```python
from build123d import *

# Parameters (mm, degrees)
SALIENTE_EXTRUIR1_DEPTH = 2
CROQUIS3_R              = 3.575
CROQUIS3_R_2            = 2.575
SALIENTE_EXTRUIR2_DEPTH = 5


with BuildPart() as part:
    # Croquis1 → Saliente-Extruir1 (new body)
    with BuildSketch(Plane(origin=(0, 0, 0), x_dir=(1, 0, 0), z_dir=(0, 1, 0))):
        with BuildLine():
            Line((-3, 13.162446581), (-4.5, 0))
            Line((-4.5, 0), (-3, -13.162446581))
            ThreePointArc((-3, -13.162446581), (0, -13.5), (3, -13.162446581))
            Line((3, -13.162446581), (4.5, 0))
            Line((4.5, 0), (3, 13.162446581))
            ThreePointArc((3, 13.162446581), (0, 13.5), (-3, 13.162446581))
        make_face()
    extrude(amount=SALIENTE_EXTRUIR1_DEPTH)

    # Croquis3 → Saliente-Extruir2 (add)
    with BuildSketch(Plane(origin=(0, 2, 0), x_dir=(1, 0, 0), z_dir=(0, 1, 0))):
        with Locations(Location((0, 0, 0), (0, 0, 270))):
            Circle(CROQUIS3_R)
        with Locations(Location((0, 0, 0), (0, 0, 270))):
            Circle(CROQUIS3_R_2, mode=Mode.SUBTRACT)
    extrude(amount=SALIENTE_EXTRUIR2_DEPTH)


solid = part.part
```
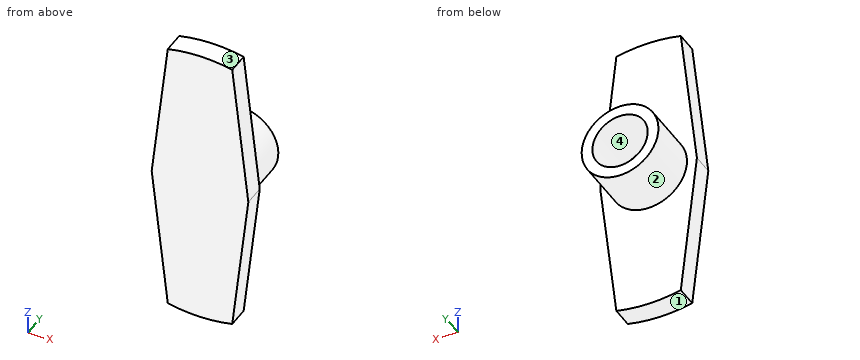
Input: part model. Units: mm. Frame: model coordinates. Face numbers are marked on the shaded views. Give positions to 0.01 mm unless a question says otherwise; leave off trailing zeros. Order: outer loops, then holes, each group sorted by start corner. A loop starts at its lowest first (then second) coordinate and runs counter-clockwise, first axis right, second up. Notation, with made-up numbers: (26, 66) - (38, 66) arc R18 cw to (38, 86) - close; hole circle Ø3 at (19, 59.25). An arc over 180 degrees is marked (long way). Use a Markdown table: item, result.
(1) Section query B-B (y = 3.25). Output: boundary loops of the cut face in (x, z) (3 decimals).
Computed values:
| item | result |
|---|---|
| outline | circle Ø7.15 at (0, 0); hole circle Ø5.15 at (0, 0) |
(2) Line query: line 1 (X direction, y = 4.3, z = 0) (3 decimals); line 2 (Y direction, x = -1.75, z = 12.5); line 3 (Z direction, x = 2, y = 3.5). Output: solid intervals per line, ascending. Write a range as from..to.
Computed values:
| item | result |
|---|---|
| line 1 | x = -3.575..-2.575, 2.575..3.575 |
| line 2 | y = 0..2 |
| line 3 | z = -2.96..-1.62, 1.62..2.96 |
(3) Section query D-D (z = 3). Output: boundary loops of the cut face in (x, y).
Computed values:
| item | result |
|---|---|
| outline | (-4.16, 0) - (4.16, 0) - (4.16, 2) - (1.94, 2) - (1.94, 7) - (-1.94, 7) - (-1.94, 2) - (-4.16, 2) - close |
(4) Draft query along Z for the marked faces 1, 2, 3 and 4. Return one class per face: released by +Z, released by -Z, zero draft, split by the parting line, or undercut.
Computed values:
| item | result |
|---|---|
| face 1 | released by -Z |
| face 2 | split by the parting line |
| face 3 | released by +Z |
| face 4 | undercut |
(5) Pin query (flat end, axial travel): pin 1 (3 mm diameter, centred on x = 3, z = 5.5, fed in from +Y); pin 2 (2 mm diameter, centred on y = 1, z = -4.5, fed in from +X). Return the tip coordinate at first contact, or that it passes through.
Computed values:
| item | result |
|---|---|
| pin 1 | stops at y = 2 |
| pin 2 | stops at x = 4.1 |
(6) Section query A-A (x = 0). Output: boundary loops of the cut face in (y, z) (3 decimals), then the cut area to 3 significant figures.
Computed values:
| item | result |
|---|---|
| outline | (0, -13.5) - (2, -13.5) - (2, -3.575) - (7, -3.575) - (7, -2.575) - (2, -2.575) - (2, 2.575) - (7, 2.575) - (7, 3.575) - (2, 3.575) - (2, 13.5) - (0, 13.5) - close |
| area | 64.0 mm2 |
(7) Section query C-C (y = 1). Output: boundary loops of the cut face in (x, z), then the cut area to 3 significant figures.
Computed values:
| item | result |
|---|---|
| outline | (-4.5, 0) - (-3, -13.16) arc R13.5 ccw to (3, -13.16) - (4.5, 0) - (3, 13.16) arc R13.5 ccw to (-3, 13.16) - close |
| area | 200 mm2 |
